from build123d import *

# Parameters (mm, degrees)
SKETCH1_R             = 56.25
SKETCH1_R_2           = 54.25
BOSS_EXTRUDE1_DEPTH   = 3
SKETCH1_R_3           = 47.5
SKETCH1_R_4           = 45.5
BOSS_EXTRUDE1_2_DEPTH = 3
SKETCH1_3_R           = 51
SKETCH1_3_R_2         = 47.5
SKETCH1_3_R_3         = 45.5
BOSS_EXTRUDE2_DEPTH   = 15
BOSS_EXTRUDE3_START   = -5
SKETCH1_4_R           = 56.25
BOSS_EXTRUDE3_DEPTH   = 5
BOSS_EXTRUDE4_DEPTH   = 5
CUT_EXTRUDE1_START    = -10
SKETCH1_5_R           = 45.5
CUT_EXTRUDE1_DEPTH    = 10
SKETCH3_R             = 2.5
CUT_EXTRUDE2_DEPTH    = 81.604745518


with BuildPart() as part:
    # Sketch1 → Boss-Extrude1 (new body)
    with BuildSketch(Plane(origin=(0, 0, 0), x_dir=(1, 0, 0), z_dir=(0, 1, 0))):
        with Locations(Location((0, 0, 0), (0, 0, 270))):
            Circle(SKETCH1_R)
        with Locations(Location((0, 0, 0), (0, 0, 270))):
            Circle(SKETCH1_R_2, mode=Mode.SUBTRACT)
    extrude(amount=BOSS_EXTRUDE1_DEPTH)



with BuildPart() as body_2:
    # Sketch1 → Boss-Extrude1 2 (new body)
    with BuildSketch(Plane(origin=(0, 0, 0), x_dir=(1, 0, 0), z_dir=(0, 1, 0))):
        with Locations(Location((0, 0, 0), (0, 0, 270))):
            Circle(SKETCH1_R_3)
        with Locations(Location((0, 0, 0), (0, 0, 270))):
            Circle(SKETCH1_R_4, mode=Mode.SUBTRACT)
    extrude(amount=BOSS_EXTRUDE1_2_DEPTH)


with BuildPart() as body_3:
    # Sketch1_3 → Boss-Extrude2 (new body)
    # profile 1 of 3: a face of its own
    with BuildSketch(Plane(origin=(0, 0, 0), x_dir=(1, 0, 0), z_dir=(0, 1, 0))):
        with Locations(Location((0, 0, 0), (0, 0, 270))):
            Circle(SKETCH1_3_R)
    # profile 2 of 3: a face of its own
    with BuildSketch(Plane(origin=(0, 0, 0), x_dir=(1, 0, 0), z_dir=(0, 1, 0))):
        with Locations(Location((0, 0, 0), (0, 0, 270))):
            Circle(SKETCH1_3_R_2)
        with Locations(Location((0, 0, 0), (0, 0, 270))):
            Circle(SKETCH1_3_R_3, mode=Mode.SUBTRACT)
    # profile 3 of 3: a face of its own
    with BuildSketch(Plane(origin=(0, 0, 0), x_dir=(1, 0, 0), z_dir=(0, 1, 0))):
        with Locations(Location((0, 0, 0), (0, 0, 270))):
            Circle(SKETCH1_3_R_3)
    extrude(amount=-BOSS_EXTRUDE2_DEPTH)


with BuildPart() as part_1:
    add(part.part)

    add(body_2.part)  # Boss-Extrude3 merges body 2

    add(body_3.part)  # Boss-Extrude3 merges body 3
    # Sketch1_4 → Boss-Extrude3 (add)
    with BuildSketch(Plane(origin=(0, 0, 0), x_dir=(1, 0, 0), z_dir=(0, 1, 0)).offset(BOSS_EXTRUDE3_START)):
        with Locations(Location((0, 0, 0), (0, 0, 270))):
            Circle(SKETCH1_4_R)
    extrude(amount=BOSS_EXTRUDE3_DEPTH)

    # Sketch2 → Boss-Extrude4 (add)
    with BuildSketch(Plane.XZ.offset(5)):
        Polygon((-2.35, -51), (-2.35, -56), (2.35, -56), (2.35, -51), (2.35, -50), (-2.35, -50), align=None)
    extrude(amount=BOSS_EXTRUDE4_DEPTH)

    # Sketch1_5 → Cut-Extrude1 (cut)
    with BuildSketch(Plane(origin=(0, 0, 0), x_dir=(1, 0, 0), z_dir=(0, 1, 0)).offset(CUT_EXTRUDE1_START)):
        with Locations(Location((0, 0, 0), (0, 0, 270))):
            Circle(SKETCH1_5_R)
    extrude(amount=CUT_EXTRUDE1_DEPTH, mode=Mode.SUBTRACT)

    # Sketch3 → Cut-Extrude2 (cut, through all)
    with BuildSketch(Plane(origin=(0, -10, 0), x_dir=(1, 0, 0), z_dir=(0, 1, 0))):
        with Locations(Location((0, -20, 0), (0, 0, 270))):
            Circle(SKETCH3_R)
    extrude(amount=-CUT_EXTRUDE2_DEPTH, mode=Mode.SUBTRACT)


solid = part_1.part
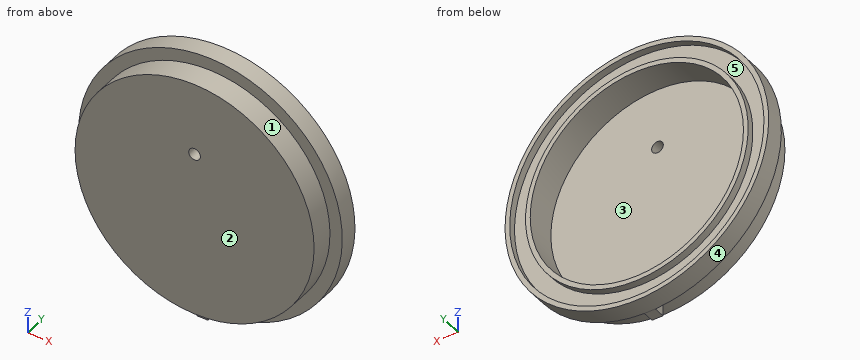
Geometry check sheet. Reference: the model listing, model coordinates, mm. Face numbers are marked on the shaded views. A direction names the side the tool comes from. Give positions to 0.01 mm unless a question says otherwise; leave off trailing zeros. Order: outer loops, then holes, each group sorted by start corner. A loop starts at its lowest first (then second) coordinate and runs counter-clockwise, first axis right, second up.
1. Sectioned sample at A-A (x = 0). Record the boundary of the cut face in (y, z), then the cut area to 4 significant figures.
Completed:
outline: (-15, -51) - (-10, -51) - (-10, -56) - (-5, -56) - (-5, -56.25) - (3, -56.25) - (3, -54.25) - (0, -54.25) - (0, -47.5) - (3, -47.5) - (3, -45.5) - (-10, -45.5) - (-10, 17.5) - (-15, 17.5) - close; (-15, 22.5) - (-10, 22.5) - (-10, 45.5) - (3, 45.5) - (3, 47.5) - (0, 47.5) - (0, 54.25) - (3, 54.25) - (3, 56.25) - (-5, 56.25) - (-5, 51) - (-15, 51) - close
area: 696.5 mm2
2. Sectioned sample at D-D (z = 0). Record the boundary of the cut face in (x, y), then the cut area to 4 significant figures.
Completed:
outline: (-56.25, -5) - (-51, -5) - (-51, -15) - (51, -15) - (51, -5) - (56.25, -5) - (56.25, 3) - (54.25, 3) - (54.25, 0) - (47.5, 0) - (47.5, 3) - (45.5, 3) - (45.5, -10) - (-45.5, -10) - (-45.5, 3) - (-47.5, 3) - (-47.5, 0) - (-54.25, 0) - (-54.25, 3) - (-56.25, 3) - close
area: 696.5 mm2
3. Depth check by flat-ended pin: pin 1 (5 mm diameter, centred on x = 0, z = -54, fed in from -Y); pin 2 (1.5 mm diameter, centred on x = -8.5, z = 29.5, fed in from +Y); pin 3 (3 mm diameter, centred on y = -11.5, z = 17.5, fed in from -X). Enter the tip coordinate at first touch or a pass-through.
Completed:
pin 1: stops at y = -10
pin 2: stops at y = -10
pin 3: stops at x = -48.43
4. Sectioned sample at C-C (y = -13.5). Record the boundary of the cut face in (x, z), then the cut area to 3 significant figures.
Completed:
outline: circle Ø102 at (0, 0); hole circle Ø5 at (0, 20)
area: 8,150 mm2
5. Draft check along X on the marked faces 1, 2 and 3. Enter one of: pulls with the +X half, pulls with the -X half, needs draft (parallel to the pull), parting line crosses it, or undercut.
Completed:
face 1: parting line crosses it
face 2: needs draft
face 3: undercut
6. Sectioned sample at B-B (z = 20). Record the boundary of the cut face in (x, y).
Completed:
outline: (-52.57, -5) - (-46.91, -5) - (-46.91, -15) - (-2.5, -15) - (-2.5, -10) - (-40.87, -10) - (-40.87, 3) - (-43.08, 3) - (-43.08, 0) - (-50.43, 0) - (-50.43, 3) - (-52.57, 3) - close; (2.5, -15) - (46.91, -15) - (46.91, -5) - (52.57, -5) - (52.57, 3) - (50.43, 3) - (50.43, 0) - (43.08, 0) - (43.08, 3) - (40.87, 3) - (40.87, -10) - (2.5, -10) - close
7. Scan lines: line 1 (X direction, y = 0.7, z = 0); line 2 (X direction, y = -5.5, z = 0); line 3 (X direction, y = -1.5, z = 0). Record each from-to range of solid material in increasing order.
Completed:
line 1: x = -56.25 to -54.25, -47.5 to -45.5, 45.5 to 47.5, 54.25 to 56.25
line 2: x = -51 to -45.5, 45.5 to 51
line 3: x = -56.25 to -45.5, 45.5 to 56.25
8. Access from +Z, -Z, +X, -X, +Y, -Y to the whole of each face (thin tool, end or side, straight path). Record for the marked faces 4 and 5.
Completed:
face 4: +Y, -Y
face 5: +Y
